from build123d import *

# Parameters (mm, degrees)
F3_DEPTH = 25
F4_R     = 7.5
F5_DEPTH = 5


# Not quite as in the source:
# - ends of sketch curves that miss each other by under 0.0002 mm in the source are joined


with BuildPart() as f1:
    # F0 (on Front) → F1 (revolve)
    with BuildSketch(Plane.XZ):
        with BuildLine():
            Line((-20.4, 8), (-25.4, 8))
            Line((-25.4, 8), (-25.4, 0))
            Line((-25.4, 0), (-12.5, 0))
            Line((-12.5, 0), (12.5, 0))
            Line((12.5, 0), (25.4, 0))
            Line((25.4, 0), (25.4, 8))
            Line((25.4, 8), (20.4, 8))
            Line((20.4, 8), (20.4, 5))
            Line((20.4, 5), (15.4, 5))
            Line((15.4, 5), (15.4, 8))
            Line((15.4, 8), (12.5, 8))
            Line((12.5, 8), (12.5, 59))
            ThreePointArc((12.5, 59), (11.0355339059, 62.5355339059), (7.5, 64))
            Line((7.5, 64), (-7.5, 64))
            ThreePointArc((-7.5, 64), (-11.0355339059, 62.5355339059), (-12.5, 59))
            Line((-12.5, 59), (-12.5, 8))
            Line((-12.5, 8), (-15.4, 8))
            Line((-15.4, 8), (-15.4, 5))
            Line((-15.4, 5), (-20.4, 5))
            Line((-20.4, 5), (-20.4, 8))
        make_face()
    revolve(axis=Axis((-6.7645025283, 0, 0), (1, 0, 0)))

    # F2 (on Front) → F3 (join, symmetric)
    with BuildSketch(Plane.XZ):
        with BuildLine():
            Line((-20.4, -10), (-15.4, -10))
            Line((-15.4, -10), (-15.4, 65.000000298))
            ThreePointArc((-15.4, 65.000000298), (-13.9355339059, 68.535534204), (-10.4, 70.000000298))
            Line((-10.4, 70.000000298), (0, 70.000000298))
            Line((0, 70.000000298), (10.4, 70.000000298))
            ThreePointArc((10.4, 70.000000298), (13.9355339059, 68.535534204), (15.4, 65.000000298))
            Line((15.4, 65.000000298), (15.4, -10))
            Line((15.4, -10), (20.4, -10))
            Line((20.4, -10), (20.4, 65.000000298))
            ThreePointArc((20.4, 65.000000298), (17.4710678407, 72.0710681387), (10.4, 75.0000003388))
            Line((10.4, 75.0000003388), (0, 75))
            Line((0, 75), (-10.4, 75))
            ThreePointArc((-10.4, 75), (-17.4710678407, 72.0710681387), (-20.4000000408, 65.000000298))
            Line((-20.4000000408, 65.000000298), (-20.4, -10))
        make_face()
    extrude(amount=F3_DEPTH, both=True)

    # F4 (on face) → F5 (join)
    with BuildSketch(Plane.XY.offset(75)):
        Circle(F4_R)
    extrude(amount=F5_DEPTH)


solid = f1.part
Design review of the part built by this model. Coordinates are the model's own, in mm. A direction names the side the tool comes from. Coordinates: 2 decimals unless noted, no trailing zeros. Write each loop counter-clockwise with the first axis right and the second up, starting at its lowest first coordinate (ties: lowest second). Pieces come first, ordered by that corner, then holes. Notation, with made-up numbers: (45, 71.5) - (100, 71.5) arc R11 cw to (100, 84.5) - close; hole circle Ø8 at (-11, -13). An arc over 180 degrees is marked (long way). One line per item, written item: value.
1) To check wall thickness, follow probe 1 along X at (y, z) = (-9, 0); probe 2 along Y at (x, z) = (19, -9.5); probe 3 along Z at (x, y) = (-1, 4.5). State the ranges of each line that lie inside material, in increasing order.
Answer sheet:
probe 1: x = -20.4 to -15.4, -12.5 to 12.5, 15.4 to 20.4
probe 2: y = -25 to 25
probe 3: z = -63.84 to 63.84, 70 to 80
2) For faces 5 (the face through (-13.97, -0.35, 68.5)), 6 (the face through (-17, 25, 39)), 7 (the face through (13.93, 7.81, -1.73)), 8 (the face through (-7.493, 0.33, 77.465)), list the 3-axis set-ups (+Z, -Z, +X, -X, +Y, -Y) from which the entire face can be reached by the end or side of a thin tool; tool diameter is ignored.
Answer sheet:
face 5: +Y, -Y
face 6: +Z, +Y
face 7: none
face 8: +Z
3) Mouldability with a two-part tool opening along Z and no side actions: class faces 1 (the face through (-17.39, -0.35, 72.15)), 2 (the face through (-18, 0, -10)), 3 (the face through (15.4, 0, 28)), 4 (the face through (-25.4, 0, 0)) as +Z half, -Z half, draft (parallel to the pull), parting line (faces both ways), or undercut.
Answer sheet:
face 1: +Z half
face 2: -Z half
face 3: undercut
face 4: draft
4) Add section C-C (z = 31.5). Give the number of separate pieces and of enclosed holes in the cut face, plus the area to 3 significant figures.
Answer sheet:
separate pieces: 3
enclosed holes: 0
area: 3,260 mm2
5) Add section A-A (x = -3). State the section outline as (y, z) points.
Answer sheet:
outline: circle Ø128 at (0, 0); (-25, 70) - (25, 70) - (25, 75) - (6.87, 75) - (6.87, 80) - (-6.87, 80) - (-6.87, 75) - (-25, 75) - close
6) Insertion check: pin 1 (12 mm diameter, centred on x = -5, z = -9.5, fed in from +Y); pin 2 (6 mm diameter, centred on y = 5, z = 59, fed in from +X); pin 3 (4 mm diameter, centred on y = -44.5, z = -43.5, fed in from -X). Each pin has a flat end and moves straight along its axis. Give the tip position at first contact, or say it passes through.
Answer sheet:
pin 1: stops at y = 63.9
pin 2: stops at x = 20.4
pin 3: stops at x = -12.35
